Here's how the part is built. I have some questions about the finished solid (model axes, mm). Coordinates: 2 decimals unless noted, no trailing zeros. Write each loop counter-clockwise with the first axis right and the second up, starting at its lowest first coordinate (ties: lowest second). Pieces come first, ordered by that corner, then holes.
Item 1: Please list where these lines run through material, in increasing order: line 1 (Y direction, x = 0, z = 3); line 2 (Y direction, x = 1, z = 8.75); line 3 (X direction, y = -1, z = 2) (3 decimals).
Item 2: I want a section at C-C (z = 8.25). Please give me the cut outline in (x, y) (1 decimal).
Item 3: I want a section at B-B (y = 0). Please give me the cut outline in (x, z) (3 decimals), and give its area (3 significant figures).
Item 4: I want a section at D-D (x = 5.25). Please give me the cut outline in (y, z).
Item 5: If we mould it in two halves opening along Y, with no side actions, what happens to faces 1 (the face through (-0.867, -3.905, 4.437)), 2 (the face through (-11.85, -26.56, 4.44)), 3 (the face through (14.385, -9, 4))? For each: pulls with the +Y half, pulls with the -Y half, needs draft (parallel to the pull), parting line crosses it, or undercut.
Item 6: I want a section at A-A (x = 0). Please give me the cut outline in (y, z), and give its area (3 significant figures).
from build123d import *

# Parameters (mm, degrees)
SKETCH_1_R      = 4
EXTRUDE_1_DEPTH = 9
CHAMFER_1_SIZE  = 5
CHAMFER_1_SIZE2 = 3
CHAMFER_2_SIZE  = 3
CHAMFER_2_SIZE2 = 5


with BuildPart() as part:
    # ｽｹｯﾁ1 → ﾎﾞｽ - 押し出し1 (new body)
    with BuildSketch(Plane.XY):
        with BuildLine():
            Line((14.385, -28.04), (-14.385, -28.04))
            Line((-14.385, -28.04), (-14.385, -5.612501624))
            Line((-14.385, -5.612501624), (-14.385, 5.612501624))
            ThreePointArc((-14.385, 5.612501624), (0, 15.34), (14.385, 5.612501624))
            Line((14.385, 5.612501624), (14.385, -5.612501624))
            Line((14.385, -5.612501624), (14.385, -28.04))
        make_face()
        Circle(SKETCH_1_R, mode=Mode.SUBTRACT)
    extrude(amount=EXTRUDE_1_DEPTH)

    # 面取り1
    chamfer_1_edges = [part.edges().sort_by_distance(p)[0] for p in [
        (14.385, -28.04, 4.5),
    ]]
    chamfer_1_side = [part.faces().sort_by_distance(p)[0] for p in [
        (0, -28.04, 4.5),
    ]]
    chamfer(chamfer_1_edges, length=CHAMFER_1_SIZE, length2=CHAMFER_1_SIZE2, reference=chamfer_1_side[0])

    # 面取り2
    chamfer_2_edges = [part.edges().sort_by_distance(p)[0] for p in [
        (-14.385, -28.04, 4.5),
    ]]
    chamfer_2_side = [part.faces().sort_by_distance(p)[0] for p in [
        (-14.385, -11.213749188, 4.5),
    ]]
    chamfer(chamfer_2_edges, length=CHAMFER_2_SIZE, length2=CHAMFER_2_SIZE2, reference=chamfer_2_side[0])


solid = part.part
Answer:
1. line 1: y = -28.04 to -4, 4 to 15.34
1. line 2: y = -28.04 to -3.87, 3.87 to 15.31
1. line 3: x = -14.385 to -3.873, 3.873 to 14.385
2. outline: (-14.4, -25) - (-9.4, -28) - (9.4, -28) - (14.4, -25) - (14.4, 5.6) arc R15.5 ccw to (-14.4, 5.6) - close; hole circle Ø8 at (0, 0)
3. outline: (-14.385, 0) - (-4, 0) - (-4, 9) - (-14.385, 9) - close; (4, 0) - (14.385, 0) - (14.385, 9) - (4, 9) - close
3. area: 187 mm2
4. outline: (-28.04, 0) - (14.42, 0) - (14.42, 9) - (-28.04, 9) - close
5. face 1: undercut
5. face 2: pulls with the -Y half
5. face 3: needs draft
6. outline: (-28.04, 0) - (-4, 0) - (-4, 9) - (-28.04, 9) - close; (4, 0) - (15.34, 0) - (15.34, 9) - (4, 9) - close
6. area: 318 mm2
